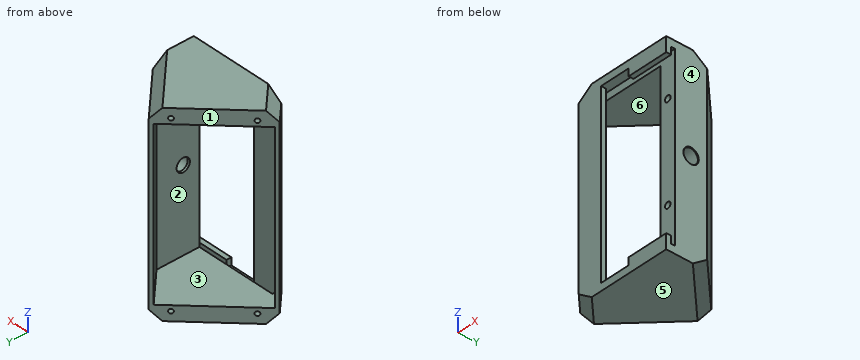
```python
from build123d import *

# Parameters (mm, degrees)
BOSS_EXTRUDE1_DEPTH  = 160.26
SKETCH2_OUTSIDE_W    = 201.942
SKETCH2_OUTSIDE_H    = 157.534
SKETCH2_OUTSIDE_W_2  = 160.26
SKETCH2_OUTSIDE_H_2  = 80
SKETCH2_OUTSIDE_W_3  = 136
SKETCH2_OUTSIDE_H_3  = 74
CUT_EXTRUDE1_DEPTH   = 156
SKETCH11_R           = 1.778
CUT_EXTRUDE8_DEPTH   = 6
BOSS_EXTRUDE14_REACH = 475.056
SKETCH19_W           = 148
SKETCH19_H           = 3.2
CUT_EXTRUDE13_DEPTH  = 79.12
SKETCH24_W           = 136
SKETCH24_H           = 4
CUT_EXTRUDE15_DEPTH  = 3
BOSS_EXTRUDE16_REACH = 475.056
CHAMFER2_SIZE        = 8.36
CUT_EXTRUDE19_REACH  = 467.887
SKETCH31_W           = 25
SKETCH31_H           = 6
SKETCH32_R           = 6.7
CUT_EXTRUDE20_DEPTH  = 10
SKETCH33_R           = 9.2
SKETCH33_R_2         = 6.7
BOSS_EXTRUDE17_DEPTH = 10
SKETCH34_R           = 9
SKETCH34_R_2         = 5.5
BOSS_EXTRUDE18_DEPTH = 2
SKETCH35_R           = 6.7
SKETCH35_R_2         = 5.95
BOSS_EXTRUDE19_DEPTH = 0.75
CHAMFER4_SIZE        = 0.375
SKETCH36_W           = 136
SKETCH36_H           = 25.327231326
SKETCH36_R           = 9.2
BOSS_EXTRUDE20_DEPTH = 10
BOSS_EXTRUDE21_DEPTH = 136
SKETCH38_R           = 2.55
CUT_EXTRUDE23_DEPTH  = 3.8
SKETCH39_R           = 1.8
CUT_EXTRUDE24_DEPTH  = 5


with BuildPart() as part:
    # Sketch1 → Boss-Extrude1 (new body)
    with BuildSketch(Plane.XY):
        Polygon((352.367164448, 53.75754858), (431.734377425, 53.75754858), (431.734377425, 87.527420593), (394.983805142, 124.277992876), (338.415262647, 67.709450381), align=None)
    extrude(amount=BOSS_EXTRUDE1_DEPTH)

    # Sketch2 outside → Cut-Extrude1 (cut)
    # profile 1 of 2: a face of its own
    with BuildSketch(Plane(origin=(135.352906133, -135.352906133, 0), x_dir=(0, 0, 1), z_dir=(-0.7071067811865476, 0.7071067811865476, 0))):
        with Locations((80.13, 335.234)):
            Rectangle(SKETCH2_OUTSIDE_W, SKETCH2_OUTSIDE_H)
        with Locations((80.13, 327.17353859)):
            Rectangle(SKETCH2_OUTSIDE_W_2, SKETCH2_OUTSIDE_H_2, mode=Mode.SUBTRACT)
    # profile 2 of 2: a face of its own
    with BuildSketch(Plane(origin=(135.352906133, -135.352906133, 0), x_dir=(0, 0, 1), z_dir=(-0.7071067811865476, 0.7071067811865476, 0))):
        with Locations((80.13, 327.17353859)):
            Rectangle(SKETCH2_OUTSIDE_W_3, SKETCH2_OUTSIDE_H_3)
    extrude(amount=-CUT_EXTRUDE1_DEPTH, mode=Mode.SUBTRACT)

    # Sketch11 → Cut-Extrude8 (cut)
    with BuildSketch(Plane(origin=(135.352906133, -135.352906133, 0), x_dir=(0, 0, 1), z_dir=(-0.7071067811865476, 0.7071067811865476, 0))):
        with Locations(Location((7.63, 353.58853859, 0), (0, 0, 270))):
            Circle(SKETCH11_R)
        with Locations(Location((7.63, 300.75853859, 0), (0, 0, 270))):
            Circle(SKETCH11_R)
        with Locations(Location((152.63, 353.58853859, 0), (0, 0, 270))):
            Circle(SKETCH11_R)
        with Locations(Location((152.63, 300.75853859, 0), (0, 0, 270))):
            Circle(SKETCH11_R)
    extrude(amount=-CUT_EXTRUDE8_DEPTH, mode=Mode.SUBTRACT)

    # Sketch17 → Boss-Extrude14 (add, up to next)
    with BuildSketch(Plane.XY.offset(12.13), mode=Mode.PRIVATE) as boss_extrude14_sk1:
        Polygon((431.734377425, 83.284779906), (431.734377425, 53.75754858), (428.734377425, 53.75754858), (428.734377425, 86.284779906), align=None)
    boss_extrude14_tool1 = extrude(boss_extrude14_sk1.sketch, amount=BOSS_EXTRUDE14_REACH, mode=Mode.PRIVATE) - part.part
    add(boss_extrude14_tool1.solids().sort_by_distance((430.210205, 69.28325, 12.13))[0])

    # Sketch19 → Cut-Extrude13 (cut)
    with BuildSketch(Plane(origin=(431.734377425, 0, 0), x_dir=(0, 0, -1), z_dir=(1, 0, 0))):
        with Locations((-80.13, 59.35754858)):
            Rectangle(SKETCH19_W, SKETCH19_H)
    extrude(amount=-CUT_EXTRUDE13_DEPTH, mode=Mode.SUBTRACT)

    # Sketch24 → Cut-Extrude15 (cut)
    with BuildSketch(Plane(origin=(431.734377425, 0, 0), x_dir=(0, 0, -1), z_dir=(1, 0, 0))):
        with Locations((-80.13, 55.75754858)):
            Rectangle(SKETCH24_W, SKETCH24_H)
    extrude(amount=-CUT_EXTRUDE15_DEPTH, mode=Mode.SUBTRACT)

    # Sketch29 → Boss-Extrude16 (add, up to next)
    with BuildSketch(Plane.XY.offset(12.13), mode=Mode.PRIVATE) as boss_extrude16_sk1:
        Polygon((356.609805135, 53.75754858), (372.609805135, 53.75754858), (372.609805135, 57.75754858), (352.609805135, 57.75754858), align=None)
    boss_extrude16_tool1 = extrude(boss_extrude16_sk1.sketch, amount=BOSS_EXTRUDE16_REACH, mode=Mode.PRIVATE) - part.part
    add(boss_extrude16_tool1.solids().sort_by_distance((363.572768, 55.831623, 12.13))[0])

    # Chamfer2
    chamfer2_edges = [part.edges().sort_by_distance(p)[0] for p in [
        (413.359091284, 105.902706735, 160.26),
        (345.391213548, 60.733499481, 160.26),
        (345.391213548, 60.733499481, 0),
        (413.359091284, 105.902706735, 0),
    ]]
    chamfer(chamfer2_edges, length=CHAMFER2_SIZE)

    # Sketch31 → Cut-Extrude19 (cut, up to next)
    with BuildSketch(Plane.XZ.offset(-53.75754858), mode=Mode.PRIVATE) as cut_extrude19_sk1:
        with Locations((385.109805135, 151.13)):
            Rectangle(SKETCH31_W, SKETCH31_H)
    cut_extrude19_tool1 = extrude(cut_extrude19_sk1.sketch, amount=-CUT_EXTRUDE19_REACH, mode=Mode.PRIVATE) & part.part
    # Sketch31 → Cut-Extrude19 (cut, up to next)
    with BuildSketch(Plane.XZ.offset(-53.75754858), mode=Mode.PRIVATE) as cut_extrude19_sk2:
        with Locations((385.109805135, 9.13)):
            Rectangle(SKETCH31_W, SKETCH31_H)
    cut_extrude19_tool2 = extrude(cut_extrude19_sk2.sketch, amount=-CUT_EXTRUDE19_REACH, mode=Mode.PRIVATE) & part.part
    add(cut_extrude19_tool1.solids().sort_by_distance((385.109805, 53.757549, 151.13))[0], mode=Mode.SUBTRACT)
    add(cut_extrude19_tool2.solids().sort_by_distance((385.109805, 53.757549, 9.13))[0], mode=Mode.SUBTRACT)

    # Sketch32 → Cut-Extrude20 (cut)
    with BuildSketch(Plane(origin=(431.734377425, 0, 0), x_dir=(0, 0, -1), z_dir=(1, 0, 0))):
        with Locations((-80.13, 74.242484587)):
            Circle(SKETCH32_R)
    extrude(amount=-CUT_EXTRUDE20_DEPTH, mode=Mode.SUBTRACT)

    # Sketch33 → Boss-Extrude17 (add)
    with BuildSketch(Plane.ZY.offset(-428.734377425)):
        with Locations(Location((80.13, 74.242484587, 0), (0, 0, 180))):
            Circle(SKETCH33_R)
        with Locations(Location((80.13, 74.242484587, 0), (0, 0, 180))):
            Circle(SKETCH33_R_2, mode=Mode.SUBTRACT)
    extrude(amount=BOSS_EXTRUDE17_DEPTH)

    # Sketch34 → Boss-Extrude18 (add)
    with BuildSketch(Plane.ZY.offset(-418.734377425)):
        with Locations((80.13, 74.242484587)):
            Circle(SKETCH34_R)
        with Locations((80.13, 74.242484587)):
            Circle(SKETCH34_R_2, mode=Mode.SUBTRACT)
    extrude(amount=-BOSS_EXTRUDE18_DEPTH)

    # Sketch35 → Boss-Extrude19 (add)
    with BuildSketch(Plane(origin=(431.734377425, 0, 0), x_dir=(0, 0, -1), z_dir=(1, 0, 0))):
        with Locations((-80.13, 74.242484587)):
            Circle(SKETCH35_R)
        with Locations((-80.13, 74.242484587)):
            Circle(SKETCH35_R_2, mode=Mode.SUBTRACT)
    extrude(amount=-BOSS_EXTRUDE19_DEPTH)

    # Chamfer4
    chamfer4_edges = [part.edges().sort_by_distance(p)[0] for p in [
        (430.984377425, 74.242484587, 86.08),
        (431.734377425, 74.242484587, 86.08),
    ]]
    chamfer(chamfer4_edges, length=CHAMFER4_SIZE - 0.0001)  # a hair under: the kernel refuses the full size

    # Sketch36 → Boss-Extrude20 (add)
    with BuildSketch(Plane.ZY.offset(-428.734377425)):
        with Locations((80.13, 73.621164243)):
            Rectangle(SKETCH36_W, SKETCH36_H)
        with Locations((80.13, 74.242484587)):
            Circle(SKETCH36_R, mode=Mode.SUBTRACT)
    extrude(amount=BOSS_EXTRUDE20_DEPTH)

    # Sketch37 → Boss-Extrude21 (add)
    with BuildSketch(Plane(origin=(0, 0, 148.13), x_dir=(-1, 0, 0), z_dir=(0, 0, -1))):
        Polygon((-418.734377425, 86.284779906), (-418.734377425, 96.284779906), (-428.734377425, 86.284779906), align=None)
    extrude(amount=BOSS_EXTRUDE21_DEPTH)

    # Sketch38 → Cut-Extrude23 (cut)
    with BuildSketch(Plane.XZ.offset(-60.95754858)):
        with Locations(Location((425.234377425, 120.13, 0), (0, 0, 270))):
            Circle(SKETCH38_R)
        with Locations(Location((425.234377425, 40.13, 0), (0, 0, 270))):
            Circle(SKETCH38_R)
    extrude(amount=-CUT_EXTRUDE23_DEPTH, mode=Mode.SUBTRACT)

    # Sketch39 → Cut-Extrude24 (cut)
    with BuildSketch(Plane.XZ.offset(-64.75754858)):
        with Locations(Location((425.234377425, 120.13, 0), (0, 0, 270))):
            Circle(SKETCH39_R)
        with Locations(Location((425.234377425, 40.13, 0), (0, 0, 270))):
            Circle(SKETCH39_R)
    extrude(amount=-CUT_EXTRUDE24_DEPTH, mode=Mode.SUBTRACT)


solid = part.part
```
Source: CAD feature listing. Evaluate the final solid. Frame: model axes, mm. Face numbers are marked on the shaded views. A direction names the side the tool comes from. Round coordinates to 2 decimals unless told otherwise and drop trailing zeros. Loops run counter-clockwise (first coordinate to the right, second up) from the corner with the lowest first, then second, coordinate; pieces in that order, holes last.
(1) Section query A-A (z = 80.13). Give the number of separate pieces and of enclosed holes in the cut face, and give its area (3 significant figures).
From the geometry:
separate pieces: 3
enclosed holes: 0
area: 502 mm2
(2) Section query C-C (x = 401.5). Output: boundary loops of the cut face in (y, z), and give its area (3 significant figures).
From the geometry:
outline: (53.76, 0) - (105.94, 0) - (117.76, 8.36) - (117.76, 151.9) - (105.94, 160.26) - (53.76, 160.26) - (53.76, 148.13) - (57.76, 148.13) - (57.76, 154.13) - (60.96, 154.13) - (60.96, 148.13) - (113.52, 148.13) - (113.52, 12.13) - (60.96, 12.13) - (60.96, 6.13) - (57.76, 6.13) - (57.76, 12.13) - (53.76, 12.13) - close
area: 1,990 mm2
(3) Section query D-D (z = 40.13). Output: boundary loops of the cut face in (x, y), and give its area (3 significant figures).
From the geometry:
outline: (338.42, 67.71) - (352.37, 53.76) - (372.61, 53.76) - (372.61, 57.76) - (352.61, 57.76) - (340.54, 69.83) - close; (392.86, 122.16) - (418.73, 96.28) - (418.73, 60.96) - (422.68, 60.96) - (422.68, 64.76) - (423.43, 64.76) - (423.43, 69.76) - (427.03, 69.76) - (427.03, 64.76) - (427.78, 64.76) - (427.78, 60.96) - (431.73, 60.96) - (431.73, 87.53) - (394.98, 124.28) - close
area: 633 mm2
(4) Access query for the marked faces 5 and 6. Directions: +Z, -Z, +X, -X, +Y, -Y. A direction counts if a zero-diameter tool reaches every point of the face in a straight line with its end or side. Return the directions, or none.
From the geometry:
face 5: -Z, +X, -X, +Y, -Y
face 6: none
(5) Material intervals for probe 1 along Z at (x, y) = (393, 60); probe 2 along Z at (x, y) = (371.5, 81); probe 3 along X at (y, z) = (63.95, 120.13), sorted ascending.
From the geometry:
probe 1: z = 0 to 6.13, 154.13 to 160.26
probe 2: z = 0 to 12.13, 148.13 to 160.26
probe 3: x = 342.17 to 346.42, 418.73 to 422.68, 427.78 to 431.73
(6) Pull-direction query (X, two-part tool) for the marked faces 1, 2, 3 and 4; classes: +X half, -X half, draft (parallel to the pull), parting line (faces both ways), or undercut.
From the geometry:
face 1: -X half
face 2: undercut
face 3: undercut
face 4: +X half
(7) Section query B-B (z = 23.5). Output: boundary loops of the cut face in (x, y), and give its area (3 significant figures).
From the geometry:
outline: (338.42, 67.71) - (352.37, 53.76) - (372.61, 53.76) - (372.61, 57.76) - (352.61, 57.76) - (340.54, 69.83) - close; (392.86, 122.16) - (418.73, 96.28) - (418.73, 60.96) - (431.73, 60.96) - (431.73, 87.53) - (394.98, 124.28) - close
area: 671 mm2
(8) Contact query for flat-ended pins moving along their axis: pin 1 Ø6.5 at (x, z) = (425.23, 120.13) entering from -Y; pin 2 Ø2 at (y, z) = (56, 150.5) entering from -X; pin 3 Ø6 at (x, z) = (367.5, 52) entering from +Y. Output: stop coordinate, or through.
From the geometry:
pin 1: stops at y = 60.96
pin 2: stops at x = 349.12
pin 3: stops at y = 57.76
